Autodesk Inventor part; units mm, degrees
ref_plane "YZ Plane" through (0, 0, 0) normal (1, 0, 0) x (0, 1, 0)
ref_plane "XZ Plane" through (0, 0, 0) normal (0, 1, 0) x (-1, 0, 0)
ref_plane "XY Plane" through (0, 0, 0) normal (0, 0, 1) x (1, 0, 0)
sketch "スケッチ1" plane through (0, 0, 0) normal (0, 1, 0) x (-1, 0, 0)
  line L0 (7.5, -7.5) -> (-7.5, -7.5)
  line L1 (-7.5, -7.5) -> (-7.5, 7.5)
  line L2 (-7.5, 7.5) -> (7.5, 7.5)
  line L3 (7.5, 7.5) -> (7.5, -7.5)
  line L4 (7.5, -7.5) -> (-7.5, 7.5) construction
  line L5 (-7.5, -7.5) -> (7.5, 7.5) construction
  line L6 (6, -6) -> (-6, -6)
  line L7 (-6, -6) -> (-6, 6)
  line L8 (-6, 6) -> (6, 6)
  line L9 (6, 6) -> (6, -6)
  point P0 (0, 0)
  dimension "d0" = 15
  dimension "d1" = 15
  dimension "d2" = 1.5
extrude "押し出し1" add sketch "スケッチ1" along normal blind 103
sketch "スケッチ2" plane through (-7.5, 0, 7.5) normal (0, 0, 1) x (1, 0, 0)
  line L0 (7.5, 0) -> (7.5, 103) construction
  line L1 (0, 103) -> (15, 103)
  line L2 (0, 0) -> (0, 103)
  line L3 (0, 51.5) -> (15, 51.5) construction
  line L4 (15, 0) -> (15, 103)
sketch "スケッチ3" plane through (7.5, 0, 7.5) normal (1, 0, 0) x (0, 0, -1)
  line L0 (7.5, 0) -> (7.5, 103) construction
  line L1 (0, 103) -> (15, 103)
  line L2 (15, 0) -> (15, 103)
  line L3 (15, 51.5) -> (0, 51.5) construction
  line L4 (0, 0) -> (0, 103)
sketch "スケッチ4" plane through (-7.5, 0, 7.5) normal (0, 0, 1) x (1, 0, 0)
  line L0 (7.5, 0) -> (7.5, 103) construction
  circle A0 centre (7.5, 7.5) radius 1.5
  line L1 (0, 0) -> (15, 0)
  circle A1 centre (7.5, 80.5) radius 1.5
  line L2 (0, 103) -> (15, 103)
  dimension "d5" = 3
  dimension "d6" = 7.5
  dimension "d13" = 3
  dimension "d23" = 22.5
extrude "押し出し2" cut sketch "スケッチ4" against normal through all
sketch "スケッチ5" plane through (7.5, 0, 7.5) normal (1, 0, 0) x (0, 0, -1)
  circle A0 centre (7.5, 20) radius 1.5
  line L0 (7.5, 0) -> (7.5, 103) construction
  line L1 (0, 0) -> (15, 0)
  circle A1 centre (10, 95.5) radius 1.5
  line L2 (0, 103) -> (15, 103)
  dimension "d9" = 3
  dimension "d10" = 20
  dimension "d15" = 3
  dimension "d16" = 7.5
  dimension "d24" = 2.5
extrude "押し出し3" cut sketch "スケッチ5" against normal through all
sketch "スケッチ6" plane through (7.5, 0, 7.5) normal (1, 0, 0) x (0, 0, -1)
  circle A0 centre (10, 95.5) radius 1.5
  line L0 (0, 103) -> (15, 103)
  circle A1 centre (7.5, 20) radius 1.5
  line L1 (0, 0) -> (15, 0)
  point P0 (7.5, 0)
  dimension "d17" = 7.5
  dimension "d18" = 83
  dimension "d19" = 103
sketch "スケッチ7" plane through (-7.5, 0, 7.5) normal (0, 0, 1) x (1, 0, 0)
  circle A0 centre (7.5, 80.5) radius 1.5
  line L0 (0, 103) -> (15, 103)
  circle A1 centre (7.5, 7.5) radius 1.5
  point P0 (7.5, 0)
  dimension "d20" = 22.5
  dimension "d21" = 95.5
equation "\"d1\" = d0"
properties part number "omu_k_jo_9" material "アルミニウム 6061-AHC"
CAD build for the part. Positions are in the model's coordinates, mm. A direction names the side the tool comes from. Give positions to 0.01 mm unless a question says otherwise; leave off trailing zeros. Write each loop counter-clockwise with the first axis right and the second up, starting at its lowest first coordinate (ties: lowest second). Pieces come first, ordered by that corner, then holes. Notation, with made-up numbers: M 72.5,-27.5 L 84.5,-27.5 A12 ccw 84.5,-10.5 Z; hole C 20,65 d11. An arc over 180 degrees is marked long. Put each result on its own line as item: value. Start each with the question number.
(1) Band-saw the part on A-A, the plane y = 80.5. Write the cut outline in (x, z), and give its area (3 significant figures).
(2) Mould opens along Y. For faces 3 (the face through (-7.5, 51, 0)), 4 (the face through (-6.74, 96.987, -2.305)), 5 (the face through (7, 0, 0)) say: +Y half, -Y half, draft (parallel to the pull), parting line (faces both ways), or undercut.
(3) Band-saw the part on B-B, the plane z = -2.5. Write the cut outline in (x, y), and give its area (3 significant figures).
(4) Band-saw the part on C-C, the plane y = 62.5. Write the cut outline in (x, z), and give its area (3 significant figures).
(5) Probe L1, parallel to Y at x = 0, z = 7.05; L2, parallel to X at y = 86, z = 0.5; L3, parallel to Y at x = -6.45, z = 0. List the from-to ranges inside material, lowest first.
(6) Band-saw the part on D-D, the plane x = -3.25. Write the cut outline in (y, z), and give its area (3 significant figures).
(7) Which spindle directions (+Z, -Z, +X, -X, +Y, -Y) get a long thin tool onto all of the face, cutting with end or side? Do faces 1 (the face through (0.806, 81.765, -6.74)), 2 (the face through (-6, 51, 0)). Say none if no direction does.
Response values:
1. outline: M -7.5,-7.5 L -1.5,-7.5 L -1.5,-6 L -6,-6 L -6,6 L -1.5,6 L -1.5,7.5 L -7.5,7.5 Z; M 1.5,-7.5 L 7.5,-7.5 L 7.5,7.5 L 1.5,7.5 L 1.5,6 L 6,6 L 6,-6 L 1.5,-6 Z
1. area: 72.0 mm2
2. face 3: draft
2. face 4: undercut
2. face 5: -Y half
3. outline: M -7.5,0 L -6,0 L -6,94 L -7.5,94 Z; M -7.5,97 L -6,97 L -6,103 L -7.5,103 Z; M 6,0 L 7.5,0 L 7.5,94 L 6,94 Z; M 6,97 L 7.5,97 L 7.5,103 L 6,103 Z
3. area: 300 mm2
4. outline: M -7.5,-7.5 L 7.5,-7.5 L 7.5,7.5 L -7.5,7.5 Z; hole M -6,-6 L 6,-6 L 6,6 L -6,6 Z
4. area: 81.0 mm2
5. L1: y = 0 to 6, 9 to 79, 82 to 103
5. L2: x = -7.5 to -6, 6 to 7.5
5. L3: y = 0 to 18.5, 21.5 to 103
6. outline: M 0,-7.5 L 103,-7.5 L 103,-6 L 0,-6 Z; M 0,6 L 103,6 L 103,7.5 L 0,7.5 Z
6. area: 309 mm2
7. face 1: +Z, -Z
7. face 2: +Y, -Y
